```python
from build123d import *

# Parameters (mm, degrees)
F0_R     = 5.065
F1_DEPTH = 8.53
F2_R     = 1
F3_R     = 1
F4_R     = 2.44
F4_R_2   = 1.54
F5_DEPTH = 2.11
F6_R     = 3.25
F6_R_2   = 2.41
F7_DEPTH = 1.03
F8_DEPTH = 4.4


with BuildPart() as f1:
    # F0 (on Top) → F1 (new body)
    with BuildSketch(Plane.XY):
        Circle(F0_R)
    extrude(amount=F1_DEPTH)

    # F2
    f2_edges = [f1.edges().sort_by_distance(p)[0] for p in [
        (-5.065, 0, 8.53),
    ]]
    fillet(f2_edges, radius=F2_R)

    # F3
    f3_edges = [f1.edges().sort_by_distance(p)[0] for p in [
        (-5.065, 0, 0),
    ]]
    fillet(f3_edges, radius=F3_R)

    # F4 (on face) → F5 (join)
    with BuildSketch(Plane.XY.offset(8.53)):
        Circle(F4_R)
        Circle(F4_R_2, mode=Mode.SUBTRACT)
    extrude(amount=F5_DEPTH)

    # F6 (on face) → F7 (join)
    with BuildSketch(Plane(origin=(0, 0, 0), x_dir=(1, 0, 0), z_dir=(0, 0, -1))):
        Circle(F6_R)
        Circle(F6_R_2, mode=Mode.SUBTRACT)
    extrude(amount=F7_DEPTH)

    # F8 (cut): a face of the model
    f8_faces = [f1.faces().sort_by_distance(p)[0] for p in [
        (0, 0, 0),
    ]]
    extrude(f8_faces, amount=-F8_DEPTH, mode=Mode.SUBTRACT)


solid = f1.part
```
Model file for the job. Use its own axes, mm. A direction names the side the tool comes from. Give positions to 0.01 mm unless a question says otherwise; leave off trailing zeros. Loops run counter-clockwise (first coordinate to the right, second up) from the corner with the lowest first, then second, coordinate; pieces in that order, holes last. Notation, with made-up numbers: M -14.75,34.25 L 42.25,34.25 A28 cw 42.25,67.25 Z; hole C 28,-0.75 d5. An arc over 180 degrees is marked long. Use one line per item in the form item = value.
Item 1: Slice it at C-C on z = 3. List the corners of the cut face in (x, y) (3 decimals), and give its area (3 significant figures).
Filled in:
outline = C 0,0 d10.13; hole C 0,0 d4.82
area = 62.3 mm^2
Item 2: Two-plate mould, pull along Y, no slides. Class faces 4 (the flat face through (-3, -2, 0)), 5 (the flat face through (0, 0, 8.53)), 6 (the cylindrical face through (4.83, 1.52, 4.22)): released by +Y, released by -Y, zero draft, split by the parting line, or undercut.
Filled in:
face_4 = zero draft
face_5 = undercut
face_6 = split by the parting line
Item 3: Drill centre lines: L1, parallel to Y at x = 0, z = 10; L2, parallel to Y at x = 0, z = 3.2 (3 decimals); L3, parallel to Z at x = -2, y = -3.25. Where is each one in solid material? Low to high.
Filled in:
L1 = -2.44 to -1.54, 1.54 to 2.44
L2 = -5.065 to -2.41, 2.41 to 5.065
L3 = 0 to 8.53
Item 4: Which spindle directions (+Z, -Z, +X, -X, +Y, -Y) get a long thin tool onto all of the face, cutting with end or side? Do faces 1 (the flat face through (0, -2, 10.64)), 2 (the flat face through (2, -2, 8.53)), 3 (the cylindrical face through (-2.579, 1.978, -0.508)). Say none if no direction does.
Filled in:
face_1 = +Z, +X, -X, +Y, -Y
face_2 = +Z
face_3 = -Z
Item 5: Flat gauge pins, fed straight in: pin 1 Ø2 at (x, y) = (3.5, -1) entering from +Z; pin 2 Ø1 at (y, z) = (1, 6.5) entering from -X; pin 3 Ø4 at (x, y) = (0, 0) entering from -Z. Where does each tip first touch, or does it go through?
Filled in:
pin_1 = 8.53
pin_2 = -5.04
pin_3 = 4.4
Item 6: Slice it at A-A on x = 0. List the corners of the cut face in (y, z) (3 decimals), and give its area (3 significant figures).
Filled in:
outline = M -5.065,1 A1 ccw -4.065,0 L -3.25,0 L -3.25,-1.03 L -2.41,-1.03 L -2.41,4.4 L 2.41,4.4 L 2.41,-1.03 L 3.25,-1.03 L 3.25,0 L 4.065,0 A1 ccw 5.065,1 L 5.065,7.53 A1 ccw 4.065,8.53 L 2.44,8.53 L 2.44,10.64 L 1.54,10.64 L 1.54,8.53 L -1.54,8.53 L -1.54,10.64 L -2.44,10.64 L -2.44,8.53 L -4.065,8.53 A1 ccw -5.065,7.53 Z
area = 69.9 mm^2
